For this review, take the finished solid that the model builds, in its own axes (mm). A direction names the side the tool comes from. Round coordinates to 2 decimals unless told otherwise and drop trailing zeros. Order: outer loops, then holes, each group sorted by start corner. A loop starts at its lowest first (then second) coordinate and runs counter-clockwise, first axis right, second up. Notation, with made-up numbers: M -17.5,87.5 L 28.5,87.5 A18 ccw 28.5,100.5 Z; hole C -25.75,6.5 d10. An arc over 180 degrees is marked long. Answer as a JSON object with one key per item and string values.
from build123d import *

# Parameters (mm, degrees)
ESQUISSE2_W             = 80
ESQUISSE2_H             = 80
BOSS_EXTRU_1_DEPTH      = 80
ESQUISSE5_W             = 80
ESQUISSE5_H             = 80
BOSS_EXTRU_2_DEPTH      = 30
ESQUISSE6_W             = 80
ESQUISSE6_H             = 80
BOSS_EXTRU_3_DEPTH      = 50
ESQUISSE7_W             = 80
ESQUISSE7_H             = 80
BOSS_EXTRU_4_DEPTH      = 50
ESQUISSE8_R             = 20
ENL_V_MAT_EXTRU_1_DEPTH = 45
ESQUISSE9_R             = 20
ENL_V_MAT_EXTRU_2_DEPTH = 65
ESQUISSE10_R            = 20
ENL_V_MAT_EXTRU_3_DEPTH = 65
ESQUISSE16_W            = 30
ESQUISSE16_H            = 30
BOSS_EXTRU_9_DEPTH      = 50
ESQUISSE17_W            = 30
ESQUISSE17_H            = 30
BOSS_EXTRU_10_DEPTH     = 50
ESQUISSE19_R            = 15
ENL_V_MAT_EXTRU_4_DEPTH = 10


with BuildPart() as part:
    # Esquisse2 → Boss.-Extru.1 (new body)
    with BuildSketch(Plane(origin=(0, 0, 0), x_dir=(1, 0, 0), z_dir=(0, 1, 0))):
        Rectangle(ESQUISSE2_W, ESQUISSE2_H)
    extrude(amount=BOSS_EXTRU_1_DEPTH)

    # Esquisse5 → Boss.-Extru.2 (add)
    with BuildSketch(Plane.ZY.offset(40)):
        with Locations((0, 40)):
            Rectangle(ESQUISSE5_W, ESQUISSE5_H)
    extrude(amount=BOSS_EXTRU_2_DEPTH)

    # Esquisse6 → Boss.-Extru.3 (add)
    with BuildSketch(Plane.XY.offset(40)):
        with Locations((0, 40)):
            Rectangle(ESQUISSE6_W, ESQUISSE6_H)
    extrude(amount=BOSS_EXTRU_3_DEPTH)

    # Esquisse7 → Boss.-Extru.4 (add)
    with BuildSketch(Plane.XZ):
        Rectangle(ESQUISSE7_W, ESQUISSE7_H)
    extrude(amount=BOSS_EXTRU_4_DEPTH)

    # Esquisse8 → Enlèv. mat.-Extru.1 (cut)
    with BuildSketch(Plane.ZY.offset(70)):
        with Locations((0, 40)):
            Circle(ESQUISSE8_R)
    extrude(amount=-ENL_V_MAT_EXTRU_1_DEPTH, mode=Mode.SUBTRACT)

    # Esquisse9 → Enlèv. mat.-Extru.2 (cut)
    with BuildSketch(Plane.XY.offset(90)):
        with Locations((0, 40)):
            Circle(ESQUISSE9_R)
    extrude(amount=-ENL_V_MAT_EXTRU_2_DEPTH, mode=Mode.SUBTRACT)

    # Esquisse10 → Enlèv. mat.-Extru.3 (cut)
    with BuildSketch(Plane.XZ.offset(50)):
        with Locations(Location((0, 0, 0), (0, 0, 270))):
            Circle(ESQUISSE10_R)
    extrude(amount=-ENL_V_MAT_EXTRU_3_DEPTH, mode=Mode.SUBTRACT)

    # Esquisse16 → Boss.-Extru.9 (add)
    with BuildSketch(Plane.XZ):
        with Locations((25, 75)):
            Rectangle(ESQUISSE16_W, ESQUISSE16_H)
    extrude(amount=BOSS_EXTRU_9_DEPTH)

    # Esquisse17 → Boss.-Extru.10 (add)
    with BuildSketch(Plane.XY.offset(40)):
        with Locations((25, -35)):
            Rectangle(ESQUISSE17_W, ESQUISSE17_H)
    extrude(amount=BOSS_EXTRU_10_DEPTH)

    # Esquisse19 → Enlèv. mat.-Extru.4 (cut)
    with BuildSketch(Plane(origin=(40, 0, 0), x_dir=(0, 0, -1), z_dir=(1, 0, 0))):
        with Locations((-73.956364881, -33.956364881)):
            Circle(ESQUISSE19_R)
        with Locations((0, 40)):
            Circle(ESQUISSE19_R)
    extrude(amount=-ENL_V_MAT_EXTRU_4_DEPTH, mode=Mode.SUBTRACT)


solid = part.part
1) For L1, parallel to Y at x = -53.5, z = 0; L2, parallel to X at y = -16, z = 0; L3, parallel to Y at x = 30, z = 46, list the stretches that pass through material, from the lowest coordinate up.
Geometry check:
{"L1": "y = 0 to 20, 60 to 80", "L2": "x = -40 to -20, 20 to 40", "L3": "y = -50 to -20, 0 to 80"}
2) Machinability: for faces 4 (the flat face through (-55, 0, -1)), 5 (the cylindrical face through (35.07, 54.872, 1.953)), 6 (the flat face through (-9, -25, 40)), 7 (the flat face through (0, 15, 0)), 8 (the flat face through (25, -10, 60)), which of the approach directions +Z, -Z, +X, -X, +Y, -Y give a long, thin tool a straight path to every point of the face, cutting with its end or side? Answer none if there is none.
Geometry check:
{"face 4": "+Z, -Z, -X, -Y", "face 5": "+X", "face 6": "-X", "face 7": "-Y", "face 8": "+X, -X"}
3) Mouldability with a two-part tool opening along Z and no side actions: class faces 1 (the flat face through (0, 40, 25)), 2 (the cylindrical face through (-47.82, 59.83, -2.6)), 3 (the flat face through (-40, -25, -1)) as +Z half, -Z half, draft (parallel to the pull), parting line (faces both ways), or undercut.
Geometry check:
{"face 1": "+Z half", "face 2": "undercut", "face 3": "draft"}
4) Add section B-B on y = 40. State the section outline as (x, z) points, and give its area (3 significant figures).
Geometry check:
{"outline": "M -70,-40 L 40,-40 L 40,-15 L 30,-15 L 30,15 L 40,15 L 40,90 L 20,90 L 20,25 L -20,25 L -20,90 L -40,90 L -40,40 L -70,40 L -70,20 L -25,20 L -25,-20 L -70,-20 Z", "area": "8,100 mm²"}
5) Add section D-D on z = 0. State the section outline as (x, y) points, and give its area (3 significant figures).
Geometry check:
{"outline": "M -70,0 L -40,0 L -40,-50 L -20,-50 L -20,15 L 20,15 L 20,-50 L 40,-50 L 40,25 L 30,25 L 30,55 L 40,55 L 40,80 L -70,80 L -70,60 L -25,60 L -25,20 L -70,20 Z", "area": "8,100 mm²"}
6) Add section A-A on z = 43. State the section outline as (x, y) points.
Geometry check:
{"outline": "M -40,0 L 40,0 L 40,80 L -40,80 Z; M 10,-50 L 40,-50 L 40,-20 L 10,-20 Z; hole C 0,40 d40"}
7) Add section C-C on x = 23. State the section outline as (y, z) points, and give its area (3 significant figures).
Geometry check:
{"outline": "M -50,-40 L 80,-40 L 80,90 L -50,90 Z; hole M -20,40 L 0,40 L 0,60 L -20,60 Z", "area": "16,500 mm²"}
8) Insertion check: P1, Ø5, axis at y = -25, z = -4, coming from the -X side; P2, Ø12, axis at x = -4.5, y = 43, coming from the +Z side; P3, Ø4, axis at x = -36, z = 72.5, coming from the -Y side. Each pin has a flat end and moves straight along its axis. Give the tip position at first contact, or say it passes through.
Geometry check:
{"P1": "stops at x = -40", "P2": "stops at z = 25", "P3": "stops at y = 0"}
